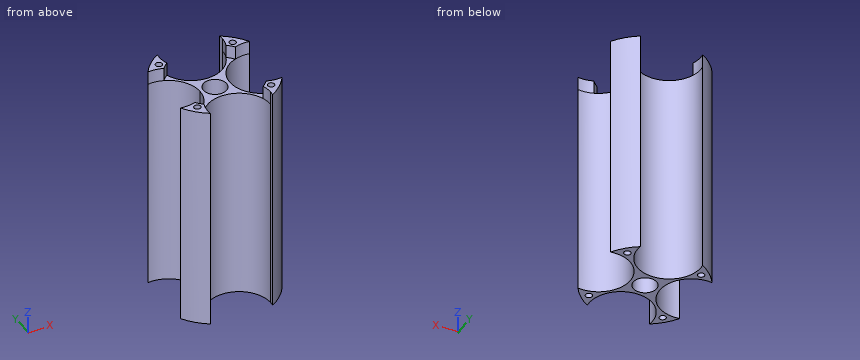
from build123d import *

# Parameters (mm, degrees)
SKETCH_1_R      = 1
SKETCH_1_R_2    = 3.5
EXTRUDE_1_DEPTH = 65
SKETCH_2_R      = 1
EXTRUDE_2_DEPTH = 4


with BuildPart() as part:
    # Эскиз1 → Бобышка-Вытянуть1 (new body)
    with BuildSketch(Plane.XY):
        with BuildLine():
            ThreePointArc((15.348214286, -9.403845928), (4.5, 0), (15.348214286, 9.403845928))
            ThreePointArc((15.348214286, 9.403845928), (12.727922061, 12.727922061), (9.403845928, 15.348214286))
            ThreePointArc((9.403845928, 15.348214286), (9.475930992, 14.675819385), (9.5, 14))
            ThreePointArc((9.5, 14), (-0.675819385, 4.524069008), (-9.403845928, 15.348214286))
            ThreePointArc((-9.403845928, 15.348214286), (-12.727922061, 12.727922061), (-15.348214286, 9.403845928))
            ThreePointArc((-15.348214286, 9.403845928), (-7.777381408, 7.178371532), (-4.5, 0))
            ThreePointArc((-4.5, 0), (-7.777381408, -7.178371532), (-15.348214286, -9.403845928))
            ThreePointArc((-15.348214286, -9.403845928), (-12.727922061, -12.727922061), (-9.403845928, -15.348214286))
            ThreePointArc((-9.403845928, -15.348214286), (-0.675819385, -4.524069008), (9.5, -14))
            ThreePointArc((9.5, -14), (9.475930992, -14.675819385), (9.403845928, -15.348214286))
            ThreePointArc((9.403845928, -15.348214286), (12.727922061, -12.727922061), (15.348214286, -9.403845928))
        make_face()
        with Locations((-11.136931804, -11.136931804)):
            Circle(SKETCH_1_R, mode=Mode.SUBTRACT)
        with Locations((11.136931804, -11.136931804)):
            Circle(SKETCH_1_R, mode=Mode.SUBTRACT)
        Circle(SKETCH_1_R_2, mode=Mode.SUBTRACT)
        with Locations((-11.136931804, 11.136931804)):
            Circle(SKETCH_1_R, mode=Mode.SUBTRACT)
        with Locations((11.136931804, 11.136931804)):
            Circle(SKETCH_1_R, mode=Mode.SUBTRACT)
    extrude(amount=EXTRUDE_1_DEPTH)

    # Эскиз2 → Бобышка-Вытянуть2 (add)
    # profile 1 of 4: a face of its own
    with BuildSketch(Plane.XY.offset(65)):
        with BuildLine():
            ThreePointArc((-9.403845928, -15.348214286), (-9.450740121, -13.033816183), (-8.936492023, -10.776785714))
            ThreePointArc((-8.936492023, -10.776785714), (-9.899494937, -9.899494937), (-10.776785714, -8.936492023))
            ThreePointArc((-10.776785714, -8.936492023), (-13.033816183, -9.450740121), (-15.348214286, -9.403845928))
            ThreePointArc((-15.348214286, -9.403845928), (-12.727922061, -12.727922061), (-9.403845928, -15.348214286))
        make_face()
        with Locations((-11.136931804, -11.136931804)):
            Circle(SKETCH_2_R, mode=Mode.SUBTRACT)
    # profile 2 of 4: a face of its own
    with BuildSketch(Plane.XY.offset(65)):
        with BuildLine():
            ThreePointArc((15.348214286, -9.403845928), (13.033816183, -9.450740121), (10.776785714, -8.936492023))
            ThreePointArc((10.776785714, -8.936492023), (9.899494937, -9.899494937), (8.936492023, -10.776785714))
            ThreePointArc((8.936492023, -10.776785714), (9.358062679, -12.363948994), (9.5, -14))
            ThreePointArc((9.5, -14), (9.475930992, -14.675819385), (9.403845928, -15.348214286))
            ThreePointArc((9.403845928, -15.348214286), (12.727922061, -12.727922061), (15.348214286, -9.403845928))
        make_face()
        with Locations((11.136931804, -11.136931804)):
            Circle(SKETCH_2_R, mode=Mode.SUBTRACT)
    # profile 3 of 4: a face of its own
    with BuildSketch(Plane.XY.offset(65)):
        with BuildLine():
            ThreePointArc((8.936492023, 10.776785714), (9.899494937, 9.899494937), (10.776785714, 8.936492023))
            ThreePointArc((10.776785714, 8.936492023), (13.033816183, 9.450740121), (15.348214286, 9.403845928))
            ThreePointArc((15.348214286, 9.403845928), (12.727922061, 12.727922061), (9.403845928, 15.348214286))
            ThreePointArc((9.403845928, 15.348214286), (9.475930992, 14.675819385), (9.5, 14))
            ThreePointArc((9.5, 14), (9.358062679, 12.363948994), (8.936492023, 10.776785714))
        make_face()
        with Locations((11.136931804, 11.136931804)):
            Circle(SKETCH_2_R, mode=Mode.SUBTRACT)
    # profile 4 of 4: a face of its own
    with BuildSketch(Plane.XY.offset(65)):
        with BuildLine():
            ThreePointArc((-10.776785714, 8.936492023), (-9.899494937, 9.899494937), (-8.936492023, 10.776785714))
            ThreePointArc((-8.936492023, 10.776785714), (-9.450740121, 13.033816183), (-9.403845928, 15.348214286))
            ThreePointArc((-9.403845928, 15.348214286), (-12.727922061, 12.727922061), (-15.348214286, 9.403845928))
            ThreePointArc((-15.348214286, 9.403845928), (-13.033816183, 9.450740121), (-10.776785714, 8.936492023))
        make_face()
        with Locations((-11.136931804, 11.136931804)):
            Circle(SKETCH_2_R, mode=Mode.SUBTRACT)
    extrude(amount=EXTRUDE_2_DEPTH)


solid = part.part
Check sheet for the modelled part. Datum: model origin and axes. Units: mm. Round coordinates to 2 decimals unless told otherwise and drop trailing zeros. Loops run counter-clockwise (first coordinate to the right, second up) from the corner with the lowest first, then second, coordinate; pieces in that order, holes last. Notation, with made-up numbers: (55, 20.25) -> (61, 20.25) arc R23 ccw to (61, 51.25) -> close; hole circle Ø1 at (-39, 44.25). An arc over 180 degrees is marked (long way). Put each result on its own line as item: value. Start each with the question number.
1. Section check C-C (z = 18.5). Enter the section's corners in (x, y).
2. Gauge pin test, flat ends, axial feed: pin 1 (11 mm diameter, centred on x = 0, y = 3, fed in from +Z); pin 2 (1.6 mm diameter, centred on x = 11.14, y = 11.14, fed in from +Z); pin 3 (1 mm diameter, centred on y = 7.5, z = 35.5, fed in from -X); pin 4 (5 mm diameter, centred on x = 7, z = 59.5, fed in from +Y). Record the tip position at first contact, or that the pin passes through.
3. Section check D-D (x = 14). Enter the section's corners in (y, z).
4. Section check B-B (y = 1). Enter the section's corners in (x, z).
5. Scan lines: probe 1 along X at (y, z) = (12, 13.5); probe 2 along Y at (x, z) = (0, 44); probe 3 along Y at (x, z) = (14, 18). Record each from-to range of solid material in increasing order.
6. Section check A-A (x = 1.5). Enter the section's corners in (y, z).
Findings:
1. outline: (-15.35, -9.4) arc R18 ccw to (-9.4, -15.35) arc R9.5 cw (long way) to (9.4, -15.35) arc R18 ccw to (15.35, -9.4) arc R9.5 cw (long way) to (15.35, 9.4) arc R18 ccw to (9.4, 15.35) arc R9.5 cw (long way) to (-9.4, 15.35) arc R18 ccw to (-15.35, 9.4) arc R9.5 cw (long way) to start; hole circle Ø2 at (-11.14, -11.14); hole circle Ø2 at (-11.14, 11.14); hole circle Ø7 at (0, 0); hole circle Ø2 at (11.14, -11.14); hole circle Ø2 at (11.14, 11.14)
2. pin 1: stops at z = 65
2. pin 2: passes through
2. pin 3: stops at x = -8.88
2. pin 4: stops at y = 15.35
3. outline: (-11.31, 0) -> (-9.5, 0) -> (-9.5, 69) -> (-11.31, 69) -> close; (9.5, 0) -> (11.31, 0) -> (11.31, 69) -> (9.5, 69) -> close
4. outline: (-4.55, 0) -> (-3.35, 0) -> (-3.35, 65) -> (-4.55, 65) -> close; (3.35, 0) -> (4.55, 0) -> (4.55, 65) -> (3.35, 65) -> close
5. probe 1: x = -13.42 to -11.64, -10.63 to -9.29, 9.29 to 10.63, 11.64 to 13.42
5. probe 2: y = -4.5 to -3.5, 3.5 to 4.5
5. probe 3: y = -11.31 to -9.5, 9.5 to 11.31
6. outline: (-4.62, 0) -> (-3.16, 0) -> (-3.16, 65) -> (-4.62, 65) -> close; (3.16, 0) -> (4.62, 0) -> (4.62, 65) -> (3.16, 65) -> close
